CAD build for the part. Positions are in the model's coordinates, mm. Round coordinates to 2 decimals unless told otherwise and drop trailing zeros. Loops run counter-clockwise (first coordinate to the right, second up) from the corner with the lowest first, then second, coordinate; pieces in that order, holes last.
Autodesk Inventor part; units mm, degrees
ref_plane "YZ Plane" through (0, 0, 0) normal (1, 0, 0) x (0, 1, 0)
ref_plane "XZ Plane" through (0, 0, 0) normal (0, 1, 0) x (-1, 0, 0)
ref_plane "XY Plane" through (0, 0, 0) normal (0, 0, 1) x (1, 0, 0)
sketch "Sketch1" plane through (0, 0, 0) normal (0, 1, 0) x (-1, 0, 0)
  circle A0 centre (0, 0) radius 37.5
  dimension "d0" = 75
extrude "Extrusion1" add sketch "Sketch1" along normal blind 5
sketch "Sketch3" plane through (0, 5, 0) normal (0, 1, 0) x (1, 0, 0)
  circle A0 centre (0, 0) radius 37.5
  line L0 (0, 32.5) -> (0, 37.5)
  line L1 (-32.5, 0) -> (-37.5, 0)
  line L2 (0, -32.5) -> (0, -37.5)
  line L3 (32.5, 0) -> (37.5, 0)
  dimension "d6" = 360
  dimension "d10" = 360
  dimension "d12" = 5
hole "Hole2" at (0, 5, -32.5) at (-32.5, 5, 0) at (0, 5, 32.5) at (32.5, 5, 0) direction (0, -1, 0) diameter 3.6 end through all
properties part number "podstava"
Item 1: Cut at D-D, the plane y = 1. Give the cut face in (x, z), plus the area to 3 significant figures.
Answers follow:
outline: circle Ø75 at (0, 0); hole circle Ø3.6 at (-32.5, 0); hole circle Ø3.6 at (0, -32.5); hole circle Ø3.6 at (0, 32.5); hole circle Ø3.6 at (32.5, 0)
area: 4,380 mm2
Item 2: Flat gauge pins, fed straight in: P1, Ø2, axis at x = -12.5, y = 2, coming from the -Z side; P2, Ø3, axis at x = 0, z = -32.5, coming from the +Y side; P3, Ø2, axis at y = 3.5, z = -23.5, coming from the +X side; P4, Ø2, axis at y = 1.5, z = -9, coming from the -X side. Where does each tip first touch, or does it go through?
Answers follow:
P1: stops at z = -35.69
P2: passes through
P3: stops at x = 30
P4: stops at x = -36.64
Item 3: Cut at C-C, the plane x = -32.5. Give the cut face in (y, z).
Answers follow:
outline: (0, -18.71) - (5, -18.71) - (5, -1.8) - (0, -1.8) - close; (0, 1.8) - (5, 1.8) - (5, 18.71) - (0, 18.71) - close
Item 4: Two-plate mould, pull along Z, no slides. Class faces 1 (the cylindrical face through (4.88, 2.46, -37.18)), 2 (the flat face through (1, 0, 1)), 3 (the cylindrical face through (-34.285, 2.465, -0.234)): released by +Z, released by -Z, zero draft, split by the parting line, or undercut.
Answers follow:
face 1: split by the parting line
face 2: zero draft
face 3: undercut
Item 5: Cut at B-B, the plane z = -32.5. Give the cut face in (x, y).
Answers follow:
outline: (-18.71, 0) - (-1.8, 0) - (-1.8, 5) - (-18.71, 5) - close; (1.8, 0) - (18.71, 0) - (18.71, 5) - (1.8, 5) - close
Item 6: Probe line 1 (Z direction, x = 0, y = 2); line 2 (X direction, y = 1.6, z = 1); line 3 (Z direction, x = 32.5, y = 1.3). List the from-to ranges inside material, lowest first.
Answers follow:
line 1: z = -37.5 to -34.3, -30.7 to 30.7, 34.3 to 37.5
line 2: x = -37.49 to -34, -31 to 31, 34 to 37.49
line 3: z = -18.71 to -1.8, 1.8 to 18.71
Item 7: Cut at A-A, the plane x = 0. Give the cut face in (y, z), plus the area to 3 significant figures.
Answers follow:
outline: (0, -37.5) - (5, -37.5) - (5, -34.3) - (0, -34.3) - close; (0, -30.7) - (5, -30.7) - (5, 30.7) - (0, 30.7) - close; (0, 34.3) - (5, 34.3) - (5, 37.5) - (0, 37.5) - close
area: 339 mm2
